The model under review builds one solid part; all positions refer to its coordinate system, in mm. Face numbers are marked on the shaded views. A direction names the side the tool comes from. Coordinates: 2 decimals unless noted, no trailing zeros. Loops run counter-clockwise (first coordinate to the right, second up) from the corner with the lowest first, then second, coordinate; pieces in that order, holes last. Notation, with made-up numbers: (20, 63.5) - (43, 63.5) arc R21 ccw to (43, 87.5) - close; hole circle Ø4 at (-11, -33). An arc over 180 degrees is marked (long way). Answer in a Markdown table with one row per item. Add a question column.
(1) For line 1 along Y through (x, z) = (38.4, 0); line 2 along Y through (x, z) = (-12, 3); line 3 along X through (y, z) = (5, 18.5), list the stretches that pass through material, from the lowest coordinate up.
(2) We need section A-A on y = 0. Write out the cut boundary in (x, z), plus the area to 3 significant figures.
(3) We need section C-C on z = 0. Write out the cut boundary in (x, y).
(4) We need section D-D on y = 10. Write out the cut boundary in (x, z), plus the area to 3 significant figures.
(5) For P1, Ø5, axis at y = -10, z = 0, coming from the -X side, flat-tipped, find the tip position at first contact; note if it passes through.
(6) Machinability: for the marked faces 1 and 2, which of the approach directions +Z, -Z, +X, -X, +Y, -Y give a long, thin tool a straight path to every point of the face, cutting with its end or side? Answer none if there is none.
(7) We need section B-B on x = 27. Write out the cut boundary in (y, z).
(8) Mouldability with a two-part tool opening along X and no side actions: class the marked faces 3, 4 and 5 as +X half, -X half, draft (parallel to the pull), parting line (faces both ways), or undercut.
from build123d import *

# Parameters (mm, degrees)
SKETCH_1_W          = 80
SKETCH_1_H          = 40
SKETCH_1_W_2        = 75
SKETCH_1_H_2        = 35
EXTRUDE_1_DEPTH     = 20
CUT_EXTRUDE_1_REACH = 82
SKETCH_3_R          = 1.6
SKETCH_3_R_2        = 5
CUT_EXTRUDE_2_REACH = 82
SKETCH_4_R          = 15
SKETCH_5_R          = 1.6
CUT_EXTRUDE_3_DEPTH = 41


with BuildPart() as part:
    # ｽｹｯﾁ1 → ﾎﾞｽ - 押し出し1 (new body, symmetric)
    with BuildSketch(Plane.XY):
        Rectangle(SKETCH_1_W, SKETCH_1_H)
        Rectangle(SKETCH_1_W_2, SKETCH_1_H_2, mode=Mode.SUBTRACT)
    extrude(amount=EXTRUDE_1_DEPTH, both=True)

    # ｽｹｯﾁ3 → ｶｯﾄ - 押し出し1 (cut, up to next)
    with BuildSketch(Plane(origin=(40, 0, 0), x_dir=(0, 0, -1), z_dir=(1, 0, 0)), mode=Mode.PRIVATE) as cut_extrude_1_sk1:
        with Locations((0, 10)):
            Circle(SKETCH_3_R)
    cut_extrude_1_tool1 = extrude(cut_extrude_1_sk1.sketch, amount=-CUT_EXTRUDE_1_REACH, mode=Mode.PRIVATE) & part.part
    add(cut_extrude_1_tool1.solids().sort_by_distance((40, 10, 0))[0], mode=Mode.SUBTRACT)
    # ｽｹｯﾁ3 → ｶｯﾄ - 押し出し1 (cut, up to next)
    with BuildSketch(Plane(origin=(40, 0, 0), x_dir=(0, 0, -1), z_dir=(1, 0, 0)), mode=Mode.PRIVATE) as cut_extrude_1_sk2:
        with Locations((10, 0)):
            Circle(SKETCH_3_R)
    cut_extrude_1_tool2 = extrude(cut_extrude_1_sk2.sketch, amount=-CUT_EXTRUDE_1_REACH, mode=Mode.PRIVATE) & part.part
    add(cut_extrude_1_tool2.solids().sort_by_distance((40, 0, -10))[0], mode=Mode.SUBTRACT)
    # ｽｹｯﾁ3 → ｶｯﾄ - 押し出し1 (cut, up to next)
    with BuildSketch(Plane(origin=(40, 0, 0), x_dir=(0, 0, -1), z_dir=(1, 0, 0)), mode=Mode.PRIVATE) as cut_extrude_1_sk3:
        with Locations((0, -10)):
            Circle(SKETCH_3_R)
    cut_extrude_1_tool3 = extrude(cut_extrude_1_sk3.sketch, amount=-CUT_EXTRUDE_1_REACH, mode=Mode.PRIVATE) & part.part
    add(cut_extrude_1_tool3.solids().sort_by_distance((40, -10, 0))[0], mode=Mode.SUBTRACT)
    # ｽｹｯﾁ3 → ｶｯﾄ - 押し出し1 (cut, up to next)
    with BuildSketch(Plane(origin=(40, 0, 0), x_dir=(0, 0, -1), z_dir=(1, 0, 0)), mode=Mode.PRIVATE) as cut_extrude_1_sk4:
        with Locations((-10, 0)):
            Circle(SKETCH_3_R)
    cut_extrude_1_tool4 = extrude(cut_extrude_1_sk4.sketch, amount=-CUT_EXTRUDE_1_REACH, mode=Mode.PRIVATE) & part.part
    add(cut_extrude_1_tool4.solids().sort_by_distance((40, 0, 10))[0], mode=Mode.SUBTRACT)
    # ｽｹｯﾁ3 → ｶｯﾄ - 押し出し1 (cut, up to next)
    with BuildSketch(Plane(origin=(40, 0, 0), x_dir=(0, 0, -1), z_dir=(1, 0, 0)), mode=Mode.PRIVATE) as cut_extrude_1_sk5:
        Circle(SKETCH_3_R_2)
    cut_extrude_1_tool5 = extrude(cut_extrude_1_sk5.sketch, amount=-CUT_EXTRUDE_1_REACH, mode=Mode.PRIVATE) & part.part
    add(cut_extrude_1_tool5.solids().sort_by_distance((40, 0, 0))[0], mode=Mode.SUBTRACT)

    # ｽｹｯﾁ4 → ｶｯﾄ - 押し出し2 (cut, up to next)
    with BuildSketch(Plane.ZY.offset(40), mode=Mode.PRIVATE) as cut_extrude_2_sk1:
        Circle(SKETCH_4_R)
    cut_extrude_2_tool1 = extrude(cut_extrude_2_sk1.sketch, amount=-CUT_EXTRUDE_2_REACH, mode=Mode.PRIVATE) & part.part
    add(cut_extrude_2_tool1.solids().sort_by_distance((-40, 0, 0))[0], mode=Mode.SUBTRACT)

    # ｽｹｯﾁ5 → ｶｯﾄ - 押し出し3 (cut, through all)
    with BuildSketch(Plane.XZ.offset(20)):
        with Locations((-32.320508076, -10)):
            Circle(SKETCH_5_R)
        with Locations((2.320508076, 10)):
            Circle(SKETCH_5_R)
    extrude(amount=-CUT_EXTRUDE_3_DEPTH, mode=Mode.SUBTRACT)


solid = part.part
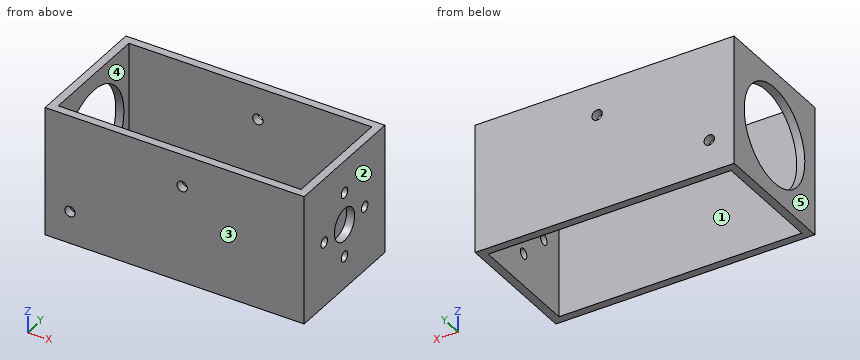
Outcome:
| question | item | result |
|---|---|---|
| 1 | line 1 | -20 to -11.6, -8.4 to -5, 5 to 8.4, 11.6 to 20 |
| 1 | line 2 | -20 to -17.5, 17.5 to 20 |
| 1 | line 3 | -40 to -37.5, 37.5 to 40 |
| 2 | outline | (-40, -20) - (-37.5, -20) - (-37.5, -15) - (-40, -15) - close; (-40, 15) - (-37.5, 15) - (-37.5, 20) - (-40, 20) - close; (37.5, -20) - (40, -20) - (40, -11.6) - (37.5, -11.6) - close; (37.5, -8.4) - (40, -8.4) - (40, -5) - (37.5, -5) - close; (37.5, 5) - (40, 5) - (40, 8.4) - (37.5, 8.4) - close; (37.5, 11.6) - (40, 11.6) - (40, 20) - (37.5, 20) - close |
| 2 | area | 84.0 mm² |
| 3 | outline | (-40, -20) - (40, -20) - (40, -11.6) - (37.5, -11.6) - (37.5, -17.5) - (-37.5, -17.5) - (-37.5, -15) - (-40, -15) - close; (-40, 15) - (-37.5, 15) - (-37.5, 17.5) - (37.5, 17.5) - (37.5, 11.6) - (40, 11.6) - (40, 20) - (-40, 20) - close; (37.5, -8.4) - (40, -8.4) - (40, -5) - (37.5, -5) - close; (37.5, 5) - (40, 5) - (40, 8.4) - (37.5, 8.4) - close |
| 4 | outline | (-40, -20) - (-37.5, -20) - (-37.5, -11.18) - (-40, -11.18) - close; (-40, 11.18) - (-37.5, 11.18) - (-37.5, 20) - (-40, 20) - close; (37.5, -20) - (40, -20) - (40, -1.6) - (37.5, -1.6) - close; (37.5, 1.6) - (40, 1.6) - (40, 20) - (37.5, 20) - close |
| 4 | area | 136 mm² |
| 5 | P1 | x = 37.5 |
| 6 | face 1 | +Z, -Z |
| 6 | face 2 | +Z, -Z, +X, +Y, -Y |
| 7 | outline | (-20, -20) - (-17.5, -20) - (-17.5, 20) - (-20, 20) - close; (17.5, -20) - (20, -20) - (20, 20) - (17.5, 20) - close |
| 8 | face 3 | draft |
| 8 | face 4 | undercut |
| 8 | face 5 | -X half |
